Read the model definition and answer for the solid it produces. Units are mm, in the model's axes. A direction names the side the tool comes from. Give positions to 0.01 mm unless a question says otherwise; leave off trailing zeros. Order: outer loops, then holes, each group sorted by start corner. A loop starts at its lowest first (then second) coordinate and runs counter-clockwise, first axis right, second up. Notation, with made-up numbers: (21.25, 55.25) -> (80.25, 55.25) arc R24 ccw to (80.25, 76.25) -> close; hole circle Ø9 at (14, -21). An arc over 180 degrees is marked (long way). Use one line per item in the form item = value.
```python
from build123d import *

# Parameters (mm, degrees)
SKETCH1_R           = 51
BOSS_EXTRUDE1_DEPTH = 11.5
SKETCH2_R           = 49.9
SKETCH2_R_2         = 4.05
BOSS_EXTRUDE2_DEPTH = 5
SKETCH3_R           = 8
CUT_EXTRUDE1_DEPTH  = 7
SKETCH4_R           = 6.5
CUT_EXTRUDE2_DEPTH  = 2.2


with BuildPart() as part:
    # Sketch1 → Boss-Extrude1 (new body)
    with BuildSketch(Plane(origin=(0, 0, 0), x_dir=(1, 0, 0), z_dir=(0, 1, 0))):
        with Locations(Location((0, 0, 0), (0, 0, 270))):
            Circle(SKETCH1_R)
        Polygon((0, 7.505553499), (-6.5, 3.75277675), (-6.5, -3.75277675), (0, -7.505553499), (6.5, -3.75277675), (6.5, 3.75277675), align=None, mode=Mode.SUBTRACT)
    extrude(amount=BOSS_EXTRUDE1_DEPTH)

    # Sketch2 → Boss-Extrude2 (add)
    with BuildSketch(Plane(origin=(0, 11.5, 0), x_dir=(1, 0, 0), z_dir=(0, 1, 0))):
        with Locations(Location((0, 0, 0), (0, 0, 270))):
            Circle(SKETCH2_R)
        with Locations(Location((0, 0, 0), (0, 0, 270))):
            Circle(SKETCH2_R_2, mode=Mode.SUBTRACT)
    extrude(amount=BOSS_EXTRUDE2_DEPTH)

    # Sketch3 → Cut-Extrude1 (cut)
    with BuildSketch(Plane.XZ):
        with Locations(Location((0, 0, 0), (0, 0, 270))):
            Circle(SKETCH3_R)
    extrude(amount=-CUT_EXTRUDE1_DEPTH, mode=Mode.SUBTRACT)

    # Sketch4 → Cut-Extrude2 (cut)
    with BuildSketch(Plane(origin=(0, 16.5, 0), x_dir=(1, 0, 0), z_dir=(0, 1, 0))):
        with Locations(Location((0, 0, 0), (0, 0, 270))):
            Circle(SKETCH4_R)
    extrude(amount=-CUT_EXTRUDE2_DEPTH, mode=Mode.SUBTRACT)


solid = part.part
```
Item 1: Determine the mould class of faces 4 (the flat face through (3, 11.5, 3)), 5 (the flat face through (-37.5, 11.5, 33.8)), 6 (the cylindrical face through (42.076, 13.965, 26.826)) for opening direction X: +X half, -X half, draft (parallel to the pull), parting line (faces both ways), or undercut.
Checks:
face_4 = undercut
face_5 = draft
face_6 = parting line
Item 2: Given pin 1 Ø3 at (y, z) = (7.5, 18) entering from -X; pin 2 Ø8 at (y, z) = (8.5, 3.5) entering from +X; pin 3 Ø2 at (y, z) = (8.5, 0.5) entering from -X, each flat-ended and moving along its own axis, determine where each tip first touches the part or whether it passes through.
Checks:
pin_1 = -48.26
pin_2 = 51
pin_3 = -51
Item 3: Straight lines are drawn through the part: L1, parallel to X at y = 15.15, z = 0; L2, parallel to X at y = 12.3, z = 0; L3, parallel to Z at x = -10.5, y = 9. For each, find the intervals that lie inside material, in ascending order. Write a range as from..to.
Checks:
L1 = -49.9..-6.5, 6.5..49.9
L2 = -49.9..-4.05, 4.05..49.9
L3 = -49.91..49.91
Item 4: Which of the six approach directions +Z, -Z, +X, -X, +Y, -Y give full straight-line access (tool end or side, diameter ignored) to faces 1 (the cylindrical face through (-3.955, 15.415, -5.158)), 2 (the flat face through (-10, 16.5, -1)), 3 (the flat face through (-6.5, 9, 0))?
Checks:
face_1 = +Y
face_2 = +Z, -Z, +X, -X, +Y
face_3 = -Y
Item 5: The part is cut by section C-C on x = -34.5. Give the vertices of the cut face in (y, z), and give its area (3 significant figures).
Checks:
outline = (0, -37.56) -> (11.5, -37.56) -> (11.5, -36.05) -> (16.5, -36.05) -> (16.5, 36.05) -> (11.5, 36.05) -> (11.5, 37.56) -> (0, 37.56) -> close
area = 1,220 mm²
Item 6: The part is cut by section A-A on z = 0. Give the vertices of the cut face in (x, y), and give its area (3 significant figures).
Checks:
outline = (-51, 0) -> (-8, 0) -> (-8, 7) -> (-6.5, 7) -> (-6.5, 11.5) -> (-4.05, 11.5) -> (-4.05, 14.3) -> (-6.5, 14.3) -> (-6.5, 16.5) -> (-49.9, 16.5) -> (-49.9, 11.5) -> (-51, 11.5) -> close; (4.05, 11.5) -> (6.5, 11.5) -> (6.5, 7) -> (8, 7) -> (8, 0) -> (51, 0) -> (51, 11.5) -> (49.9, 11.5) -> (49.9, 16.5) -> (6.5, 16.5) -> (6.5, 14.3) -> (4.05, 14.3) -> close
area = 1,450 mm²
Item 7: The part is cut by section D-D on z = 35. Give the vertices of the cut face in (x, y).
Checks:
outline = (-37.09, 0) -> (37.09, 0) -> (37.09, 11.5) -> (35.57, 11.5) -> (35.57, 16.5) -> (-35.57, 16.5) -> (-35.57, 11.5) -> (-37.09, 11.5) -> close
Item 8: The part is cut by section B-B on y = 2. Give the vertices of the cut face in (x, z).
Checks:
outline = circle Ø102 at (0, 0); hole circle Ø16 at (0, 0)
